Check sheet for the modelled part. Datum: model origin and axes. Units: mm. Face numbers are marked on the shaded views. A direction names the side the tool comes from. Coordinates: 2 decimals unless noted, no trailing zeros. Order: outer loops, then holes, each group sorted by start corner. A loop starts at its lowest first (then second) coordinate and runs counter-clockwise, first axis right, second up.
1. Cross-section at A-A (y = 2.5). Enter the section's corners in (x, z).
2. Thickness scan on line 1 (Z direction, x = 0, y = -2.55); line 2 (Y direction, x = 1.75, z = 2.25). Record the ranges inside material, lowest first.
3. Draft check along X on the marked faces 1, 2 and 3. Enter one of: released by +X, released by -X, zero draft, split by the parting line, or undercut.
4. Gauge pin test, flat ends, axial feed: pin 1 Ø2.5 at (x, z) = (0, 0) entering from -Y; pin 2 Ø2 at (x, y) = (-1, 21.5) entering from +Z; pin 3 Ø2 at (y, z) = (0.5, 2) entering from +X. Record the tip position at first contact, or that the pin passes through.
5. Set-up check for the marked faces 4, 5 and 6: record each of +Z, -Z, +X, -X, +Y, -Y from which the full face is reachable in a straight line by a thin tool's end or side.
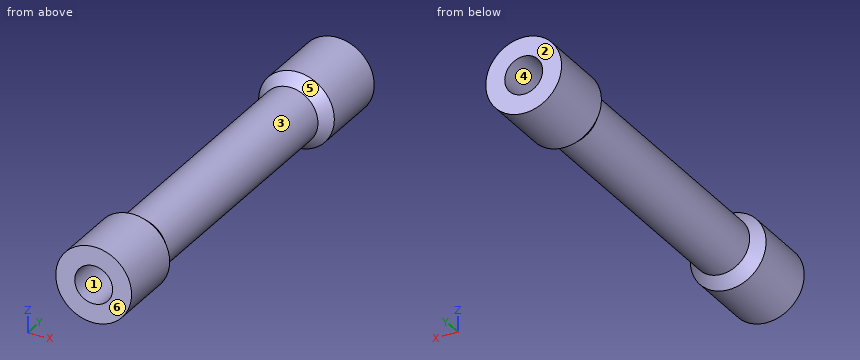
Autodesk Fusion 360 part; units mm, degrees
sketch "Sketch2" plane through (0, 30, 0) normal (0, 1, 0) x (-1, 0, 0)
  circle A0 centre (0, 0) radius 3
  circle A1 centre (0, 0) radius 3
ref_plane "WorkPlane1" through (0, 23.5, 0) normal (0, 1, 0) x (-1, 0, 0)
ref_plane "WorkPlane2" through (0, 22.5, 0) normal (0, 1, 0) x (-1, 0, 0)
sketch "Sketch3" plane through (0, 22.5, 0) normal (0, 1, 0) x (1, 0, 0)
  circle A0 centre (0, 0) radius 2.25
  dimension "d12" = 4.5
sketch "Sketch4" plane through (0, 23.5, 0) normal (0, 1, 0) x (1, 0, 0)
  circle A0 centre (0, 0) radius 3
  dimension "d13" = 6
extrude "Extrude2" add sketch "Sketch2" against normal blind 6.5
loft "Loft1" add profiles "Sketch4", "Sketch3" section 1 section 2
extrude "Extrude3" add 1 faces at (-0.1619, 22.5, 0.6982) along direction (0, -1, 0) blind 21.75
ref_plane "WorkPlane3" through (0, -0.25, 0) normal (0, -1, 0) x (0, 0, -1)
sketch "Sketch5" plane through (0, -0.25, 0) normal (0, -1, 0) x (1, 0, 0)
  circle A0 centre (0, 0) radius 3
  dimension "d19" = 6
loft "Loft2" add profiles "Sketch5" section 1 face at (-0.1619, 0.75, 0.6982) section 2
extrude "Extrude4" add 1 faces at (-1.1591, -0.25, 0.5829) along direction (0, -1, 0) blind 5.5
extrude "Extrude5" cut 1 faces at (1.1591, 30, 0.5829) along direction (0, -1, 0) blind 0.75
hole "Hole3" at (0, 29.25, 0) direction (0, -1, 0) diameter 3 depth 5 tip angle 118
hole "Hole4" at (0, -5.75, 0) direction (0, 1, 0) diameter 3 depth 5 tip angle 118
thread "Thread3"
thread "Thread4"
Data:
1. outline: circle Ø4.5 at (0, 0)
2. line 1: z = -3 to -1.5, 1.5 to 3
2. line 2: y = -5.75 to -0.05, 23.3 to 29.25
3. face 1: undercut
3. face 2: zero draft
3. face 3: split by the parting line
4. pin 1: stops at y = -0.6
4. pin 2: stops at z = 2.25
4. pin 3: stops at x = 2.68
5. face 4: +Y
5. face 5: none
5. face 6: +Z, -Z, +X, -X, -Y
